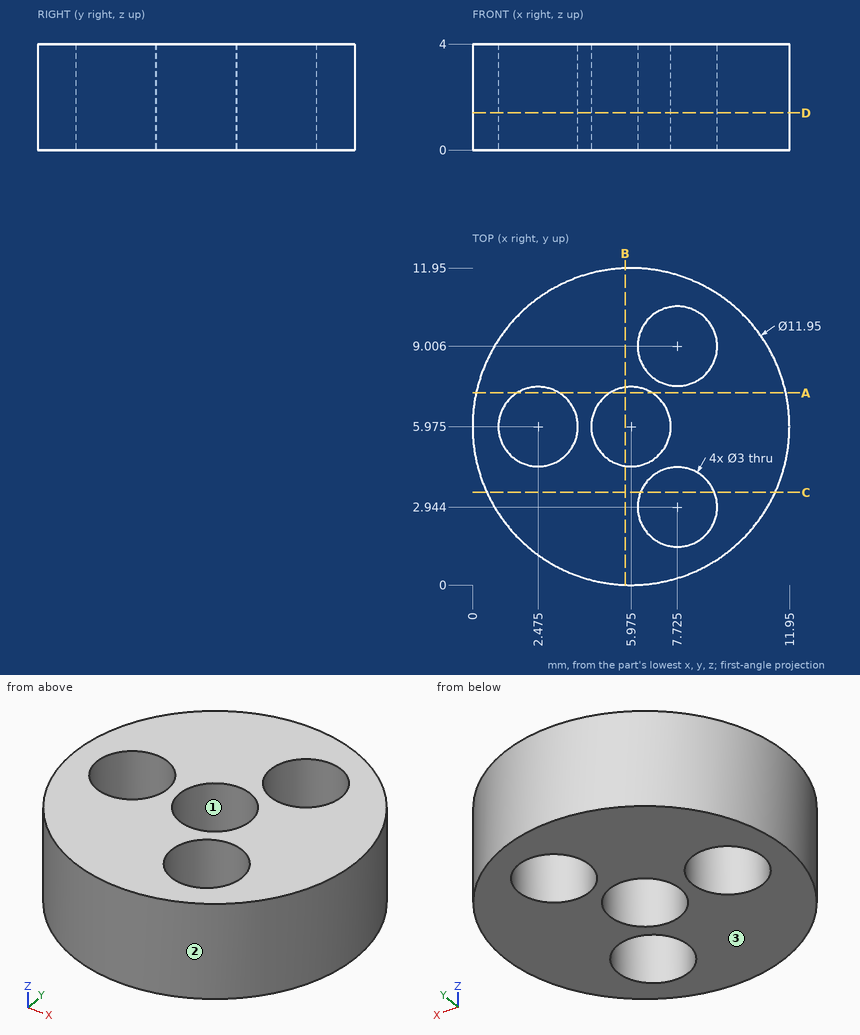
Check sheet for the drawn part. Datum: minimum x, y, z corner. Units: mm. Round coordinates to 2 decimals unless told otherwise and drop trailing zeros. Loops run counter-clockwise (first coordinate to the right, second up) from the corner with the lowest first, then second, coordinate; pieces in that order, holes last. Notation, with made-up numbers: (-26.5, 7) -> (-8.5, 7) arc R15 ccw to (-8.5, 35) -> close; hole circle Ø6 at (5, 77.5). An arc over 180 degrees is marked (long way). Put each result on its own line as item: value. Start each with the question number.
1. Section check A-A (y = 7.25). Enter the section's corners in (x, z) (1 decimal).
2. Gauge pin test, flat ends, axial feed: pin 1 (2.5 mm diameter, centred on x = 7.72, y = 9.01, fed in from -Z); pin 2 (2 mm diameter, centred on y = 10.5, z = 3, fed in from +X); pin 3 (2 mm diameter, centred on y = 1.5, z = 3, fed in from -X); pin 4 (1.5 mm diameter, centred on x = 7.5, z = 1.5, fed in from -Y). Record the tip position at first contact, or that the pin passes through.
3. Draft check along Y on the marked faces 1, 2 and 3. Enter one of: +Y half, -Y half, draft (parallel to the pull), parting line (faces both ways), or undercut.
4. Section check D-D (z = 1.4). Enter the section's corners in (x, y) (3 decimals), plus the area to 3 significant figures.
5. Section check C-C (y = 3.5). Enter the section's corners in (x, z), plus the area to 3 significant figures.
6. Section check B-B (x = 5.75). Enter the section's corners in (y, z), plus the area to 3 significant figures.
7. Scan lines: probe 1 along X at (y, z) = (6, 0.95) (3 decimals); probe 2 along Y at (x, z) = (6, 1.4) (3 decimals); probe 3 along Y at (x, z) = (8.5, 1.6). Record each from-to range of solid material in increasing order.
Findings:
1. outline: (0.1, 0) -> (1.7, 0) -> (1.7, 4) -> (0.1, 4) -> close; (3.3, 0) -> (5.2, 0) -> (5.2, 4) -> (3.3, 4) -> close; (6.8, 0) -> (11.8, 0) -> (11.8, 4) -> (6.8, 4) -> close
2. pin 1: passes through
2. pin 2: stops at x = 10.8
2. pin 3: stops at x = 1.11
2. pin 4: stops at y = 0.05
3. face 1: undercut
3. face 2: parting line
3. face 3: draft
4. outline: circle Ø11.95 at (5.975, 5.975); hole circle Ø3 at (2.475, 5.975); hole circle Ø3 at (5.975, 5.975); hole circle Ø3 at (7.725, 2.944); hole circle Ø3 at (7.725, 9.006)
4. area: 83.9 mm^2
5. outline: (0.54, 0) -> (6.33, 0) -> (6.33, 4) -> (0.54, 4) -> close; (9.12, 0) -> (11.41, 0) -> (11.41, 4) -> (9.12, 4) -> close
5. area: 32.4 mm^2
6. outline: (0, 0) -> (4.49, 0) -> (4.49, 4) -> (0, 4) -> close; (7.46, 0) -> (11.95, 0) -> (11.95, 4) -> (7.46, 4) -> close
6. area: 35.9 mm^2
7. probe 1: x = 0 to 0.975, 3.975 to 4.475, 7.475 to 11.95
7. probe 2: y = 0 to 4.475, 7.475 to 11.95
7. probe 3: y = 0.56 to 1.66, 4.23 to 7.72, 10.29 to 11.39
